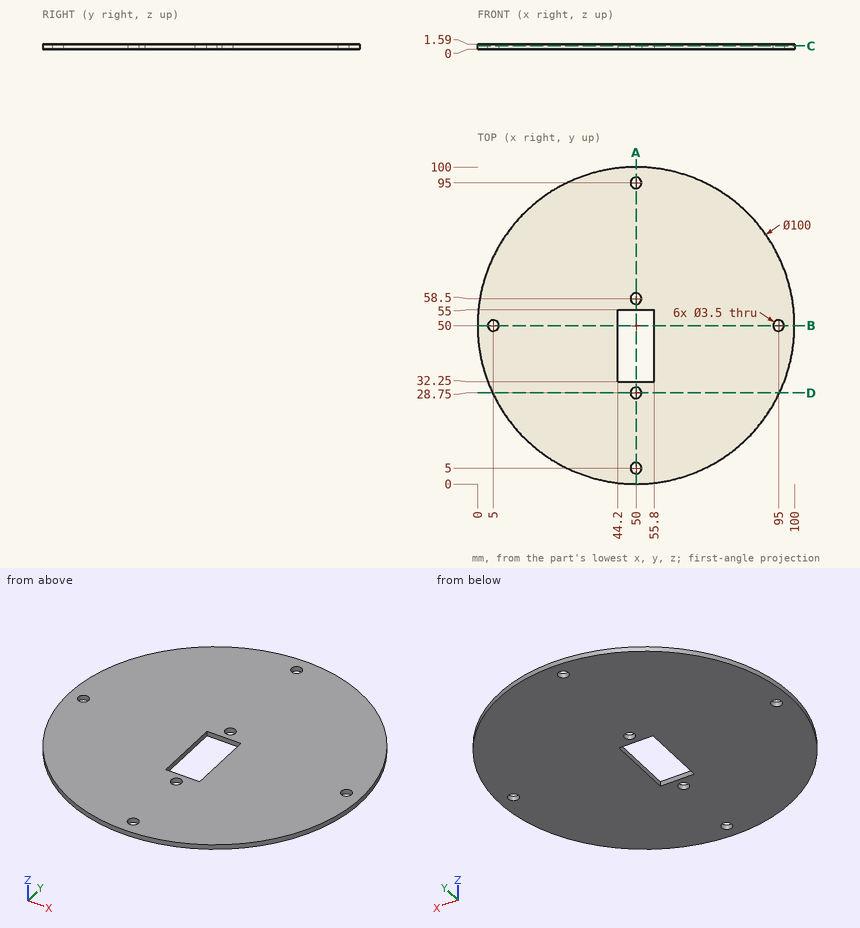
Print and shaded views of the part. All mm, measured from the part's lowest x, y and z. Give positions to 0.01 mm unless a question says otherwise; leave off trailing zeros. Loops run counter-clockwise (first coordinate to the right, second up) from the corner with the lowest first, then second, coordinate; pieces in that order, holes last. Notation, with made-up numbers: (19, -24.5) -> (57, -24.5) arc R12 ccw to (57, -9.5) -> close; hole circle Ø6 at (72.5, -3.5). An arc over 180 degrees is marked (long way). Use a Markdown table: item, result.
1. Slice it at B-B (y = 50). List the corners of the cut face in (x, z), plus the area to 3 significant figures.
Check result:
| item | result |
|---|---|
| outline | (0, 0) -> (3.25, 0) -> (3.25, 1.59) -> (0, 1.59) -> close; (6.75, 0) -> (44.2, 0) -> (44.2, 1.59) -> (6.75, 1.59) -> close; (55.8, 0) -> (93.25, 0) -> (93.25, 1.59) -> (55.8, 1.59) -> close; (96.75, 0) -> (100, 0) -> (100, 1.59) -> (96.75, 1.59) -> close |
| area | 129 mm^2 |
2. Slice it at C-C (z = 1). List the corners of the cut face in (x, y).
Check result:
| item | result |
|---|---|
| outline | circle Ø100 at (50, 50); hole circle Ø3.5 at (5, 50); hole (44.2, 32.25) -> (55.8, 32.25) -> (55.8, 55) -> (44.2, 55) -> close; hole circle Ø3.5 at (50, 5); hole circle Ø3.5 at (50, 28.75); hole circle Ø3.5 at (50, 58.5); hole circle Ø3.5 at (50, 95); hole circle Ø3.5 at (95, 50) |
3. Slice it at D-D (y = 28.75). List the corners of the cut face in (x, z), plus the area to 3 significant figures.
Check result:
| item | result |
|---|---|
| outline | (4.74, 0) -> (48.25, 0) -> (48.25, 1.59) -> (4.74, 1.59) -> close; (51.75, 0) -> (95.26, 0) -> (95.26, 1.59) -> (51.75, 1.59) -> close |
| area | 138 mm^2 |
4. Slice it at A-A (x = 50). List the corners of the cut face in (y, z).
Check result:
| item | result |
|---|---|
| outline | (0, 0) -> (3.25, 0) -> (3.25, 1.59) -> (0, 1.59) -> close; (6.75, 0) -> (27, 0) -> (27, 1.59) -> (6.75, 1.59) -> close; (30.5, 0) -> (32.25, 0) -> (32.25, 1.59) -> (30.5, 1.59) -> close; (55, 0) -> (56.75, 0) -> (56.75, 1.59) -> (55, 1.59) -> close; (60.25, 0) -> (93.25, 0) -> (93.25, 1.59) -> (60.25, 1.59) -> close; (96.75, 0) -> (100, 0) -> (100, 1.59) -> (96.75, 1.59) -> close |
5. Wall check: L1, parallel to Y at x = 50, z = 0.4; L2, parallel to X at y = 95, z = 1.05. Give the ranges that are in metal, low to high. Write a range as [from, to].
Check result:
| item | result |
|---|---|
| L1 | y = [0, 3.25], [6.75, 27], [30.5, 32.25], [55, 56.75], [60.25, 93.25], [96.75, 100] |
| L2 | x = [28.21, 48.25], [51.75, 71.79] |
6. Flat gauge pins, fed straight in: pin 1 (4 mm diameter, centred on x = 50, y = 5, fed in from +Z); pin 2 (3 mm diameter, centred on x = 95, y = 50, fed in from -Z). Where does each tip first touch, or does it go through?
Check result:
| item | result |
|---|---|
| pin 1 | stops at z = 1.59 |
| pin 2 | passes through |
